Job drawing, mm, ordinate dimensions from the low corner. One solid piece. A direction names the side the tool comes from. Give positions to 0.01 mm unless a question says otherwise; leave off trailing zeros. Write each loop counter-clockwise with the first axis right and the second up, starting at its lowest first coordinate (ties: lowest second). Pieces come first, ordered by that corner, then holes. Notation, with made-up numbers: M 64.5,54.25 L 89.5,54.25 A27 ccw 89.5,85.25 Z; hole C -20.5,50 d7. An arc over 180 degrees is marked long. Use CSV: the item, a comma, the result in double quotes. Start each with the question number.
Item 1: Cut at A-A (x = 18.55). List the corners of the cut face in (y, z).
Item 2: Cut at D-D (x = 8). List the corners of the cut face in (y, z).
Item 3: Pin check, flat tips, straight feed: pin 1 (1.2 mm diameter, centred on y = 3, z = 6, fed in from -X); pin 2 (3 mm diameter, centred on x = 12.5, z = 13.5, fed in from +Y); pin 3 (3 mm diameter, centred on x = 33, y = 16.5, fed in from +Z). Stop position of each tip, or through.
Item 4: Cut at C-C (z = 6.5). List the corners of the cut face in (x, y).
Item 5: Drill centre lines: line 1 (Y direction, x = 18.55, z = 4.1); line 2 (Z direction, x = 13, y = 21); line 3 (Y direction, x = 18.55, z = 6.6) (1 decimal). Where is each one in solid material? Low to high. Write a range as [from, to].
Item 6: Which spindle directions (+Z, -Z, +X, -X, +Y, -Y) get a long thin tool onto all of the face, cutting with end or side? Do the marked faces 1, 2 and 3. Say none if no direction does.
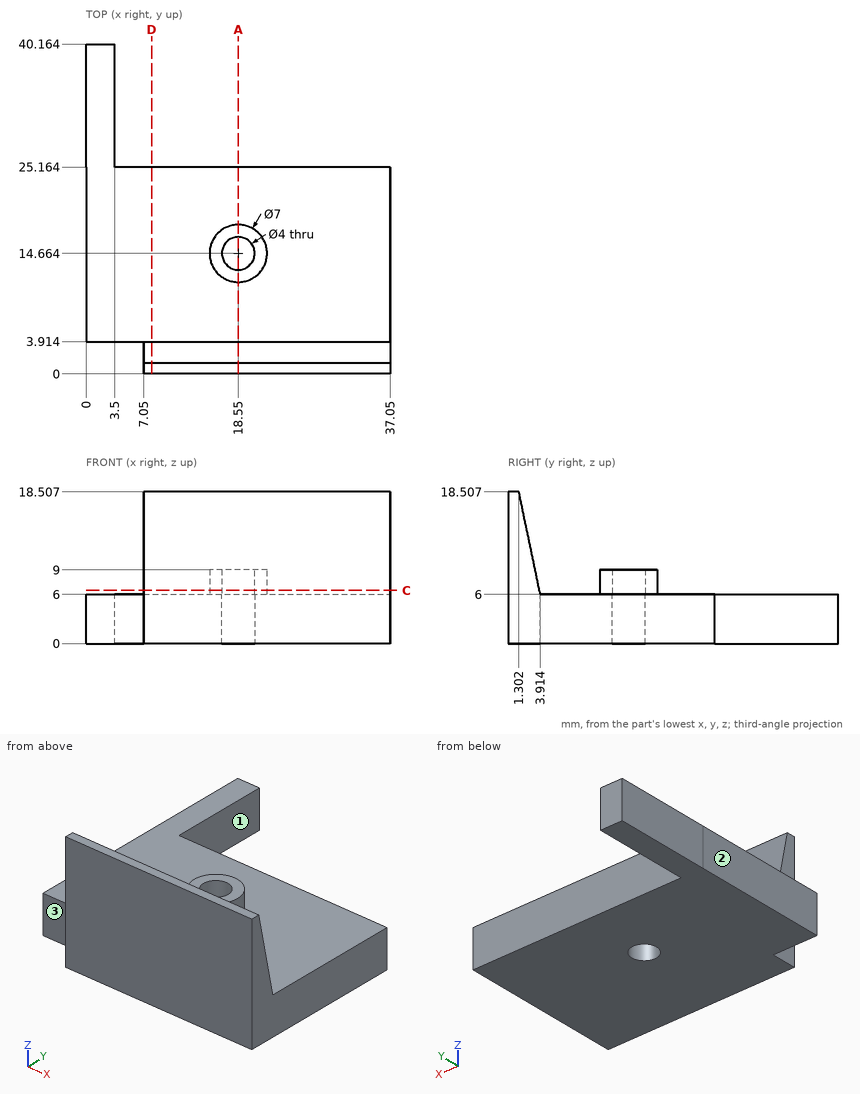
Worked answers:
1,outline,"M 0,0 L 12.66,0 L 12.66,9 L 11.16,9 L 11.16,6 L 3.91,6 L 1.3,18.51 L 0,18.51 Z; M 16.66,0 L 25.16,0 L 25.16,6 L 18.16,6 L 18.16,9 L 16.66,9 Z"
2,outline,"M 0,0 L 25.16,0 L 25.16,6 L 3.91,6 L 1.3,18.51 L 0,18.51 Z"
3,pin 1,"stops at x = 7.05"
3,pin 2,"stops at y = 2.66"
3,pin 3,"stops at z = 6"
4,outline,"M 7.05,0 L 37.05,0 L 37.05,3.81 L 7.05,3.81 Z; C 18.55,14.66 d7; hole C 18.55,14.66 d4"
5,line 1,"y = [0, 12.66], [16.66, 25.16]"
5,line 2,"z = [0, 6]"
5,line 3,"y = [0, 3.8], [11.2, 12.7], [16.7, 18.2]"
6,face 1,"+Z, -Z, +X, +Y"
6,face 2,"+Z, -Z, -X, +Y, -Y"
6,face 3,"+Z, -Z, -X, -Y"
